Check sheet for the modelled part. Datum: model origin and axes. Units: mm. Face numbers are marked on the shaded views. A direction names the side the tool comes from. Coordinates: 2 decimals unless noted, no trailing zeros. Write each loop counter-clockwise with the first axis right and the second up, starting at its lowest first coordinate (ties: lowest second). Pieces come first, ordered by that corner, then holes. Notation, with made-up numbers: (84, -8.5) - (99, -8.5) arc R30 cw to (99, 25.5) - close; hole circle Ø5 at (-5.75, 82.25). An arc over 180 degrees is marked (long way). Write each question's results on one line, items separated by ' | '.
from build123d import *

# Parameters (mm, degrees)
SKETCH_2_W                  = 1.5
SKETCH_2_H                  = 15
PATTERN_LINEAR_1_COUNT      = 3
PATTERN_LINEAR_1_PITCH      = 7.071067812
PATTERN_LINEAR_1_COUNT_DIR2 = 3
PATTERN_LINEAR_1_PITCH_DIR2 = 7.071067812


with BuildPart() as part:
    # Sketch 1 → Revolve 1 (revolve)
    with BuildSketch(Plane.XY, mode=Mode.PRIVATE) as revolve_1_sk:
        Polygon((0, 4.5), (12, 4.5), (12, 0), (11, 0), (11, -3), (0, -3), align=None)
    revolve(revolve_1_sk.sketch.rotate(Axis((0, -3, 0), (0, 1, 0)), 270), axis=Axis((0, -3, 0), (0, 1, 0)))

    # Sketch 2 → Cut-Revolve 1 (revolve, cut)
    with BuildSketch(Plane.XY, mode=Mode.PRIVATE) as cut_revolve_1_sk:
        with Locations((0.75, -3)):
            Rectangle(SKETCH_2_W, SKETCH_2_H)
    revolve(cut_revolve_1_sk.sketch.rotate(Axis((0, -10.5, 0), (0, 1, 0)), 270), axis=Axis((0, -10.5, 0), (0, 1, 0)), mode=Mode.SUBTRACT)

    # Sketch 3 → Cut-Revolve 2 (revolve, cut)
    with BuildSketch(Plane.XY, mode=Mode.PRIVATE) as cut_revolve_2_sk:
        Polygon((10, 4.5), (11, 4.5), (10.7835, 4.2835), (10.7835, 1.202353936), (10, 0.75), align=None)
    cut_revolve_2 = revolve(cut_revolve_2_sk.sketch.rotate(Axis((10, 0.75, 0), (0, 1, 0)), 270), axis=Axis((10, 0.75, 0), (0, 1, 0)), mode=Mode.SUBTRACT)

    # Pattern Linear 1: Cut-Revolve 2 3 × 3, 1 skipped
    with Locations(*[Vector(-0.7071067811865475, 0, -0.7071067811865477) * (i * PATTERN_LINEAR_1_PITCH) + Vector(-0.7071067811865477, 0, 0.7071067811865475) * (j * PATTERN_LINEAR_1_PITCH_DIR2) for i in range(PATTERN_LINEAR_1_COUNT) for j in range(PATTERN_LINEAR_1_COUNT_DIR2) if (i, j) not in ((0, 0), (1, 1))]):
        add(cut_revolve_2, mode=Mode.SUBTRACT)


solid = part.part
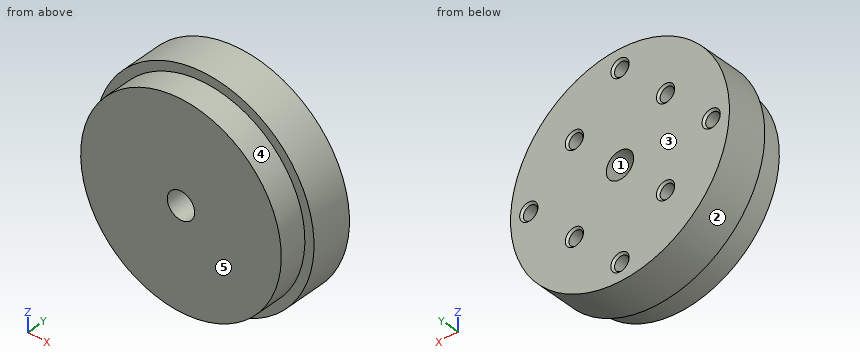
1. Sectioned sample at A-A (y = 3). Give the number of separate pieces and of enclosed holes in the cut face, then the cut area to 3 significant figures.
Values follow:
separate pieces: 1 | enclosed holes: 9 | area: 430 mm^2
2. Material ranges on L1, parallel to X at y = 3.25, z = 0; L2, parallel to X at y = 3.5, z = 5.25; L3, parallel to X at y = 3.25, z = 5, recorded low to high. Write a range as [from, to].
Values follow:
L1: x = [-12, -10.78], [-9.22, -1.5], [1.5, 9.22], [10.78, 12] | L2: x = [-10.79, -5.74], [-4.26, 4.26], [5.74, 10.79] | L3: x = [-10.91, -5.78], [-4.22, 4.22], [5.78, 10.91]
3. Sectioned sample at B-B (x = 8.5). Record the cut outline in (y, z).
Values follow:
outline: (-3, -6.98) - (0, -6.98) - (0, -8.47) - (4.5, -8.47) - (4.5, 8.47) - (0, 8.47) - (0, 6.98) - (-3, 6.98) - close
4. Draft check along X on the marked faces 1, 2 and 3. Enter one of: pulls with the +X half, pulls with the -X half, needs draft (parallel to the pull), parting line crosses it, or undercut.
Values follow:
face 1: undercut | face 2: parting line crosses it | face 3: needs draft
5. Go/stop test with flat-tipped pins: pin 1 (1.5 mm diameter, centred on y = 3.5, z = -2, fed in from -X); pin 2 (3 mm diameter, centred on y = 1, z = -6.5, fed in from +X); pin 3 (1.5 mm diameter, centred on x = -6, y = -1.5, fed in from +Z). Record where each tip stops, or that it passes through.
Values follow:
pin 1: stops at x = -11.93 | pin 2: stops at x = 10.91 | pin 3: stops at z = 9.67
6. Sectioned sample at C-C (z = 7.75). Record the cut outline in (x, y).
Values follow:
outline: (-9.16, 0) - (-7.81, 0) - (-7.81, -3) - (7.81, -3) - (7.81, 0) - (9.16, 0) - (9.16, 4.5) - (-9.16, 4.5) - close
7. Access from +Z, -Z, +X, -X, +Y, -Y to the whole of each face (thin tool, end or side, straight path). Record for the marked faces 4 and 5.
Values follow:
face 4: -Y | face 5: +Z, -Z, +X, -X, -Y
